Could you check a few things on this model? Use its own coordinates, in mm. A direction names the side the tool comes from. Round coordinates to 2 decimals unless told otherwise and drop trailing zeros. Loops run counter-clockwise (first coordinate to the right, second up) from the corner with the lowest first, then second, coordinate; pieces in that order, holes last. Notation, with made-up numbers: (61.5, -12) -> (113.5, -12) arc R8 cw to (113.5, 2) -> close; hole circle Ø3 at (77.5, -33.5). An arc over 180 degrees is marked (long way). One line per item, written item: value.
```python
from build123d import *

# Parameters (mm, degrees)
F0_W     = 50
F0_H     = 160
F0_R     = 3.25
F1_DEPTH = 5
F0_W_2   = 60
F2_DEPTH = 25


# Not quite as in the source:
# - a feature names something its author has since deleted; it is built from what else it names


with BuildPart() as f1:
    # F0 (on Front) → F1 (new body)
    with BuildSketch(Plane.XZ):
        with Locations((-52.5, 0)):
            Rectangle(F0_W, F0_H)
        with Locations((-47.5, -60)):
            Circle(F0_R, mode=Mode.SUBTRACT)
        with Locations((-47.5, 60)):
            Circle(F0_R, mode=Mode.SUBTRACT)
    extrude(amount=F1_DEPTH)



with BuildPart() as f1b:
    # F0 (on Front) → F1, piece 2 (new body)
    with BuildSketch(Plane.XZ):
        with Locations((57.5, 0)):
            Rectangle(F0_W, F0_H)
        with Locations((47.5, -60)):
            Circle(F0_R, mode=Mode.SUBTRACT)
        with Locations((47.5, 60)):
            Circle(F0_R, mode=Mode.SUBTRACT)
    extrude(amount=F1_DEPTH)


with BuildPart() as f1_1:
    add(f1.part)

    add(f1b.part)  # F2 merges F1b
    # F0 (on Front) → F2 (join)
    with BuildSketch(Plane.XZ):
        with Locations((2.5, 0)):
            Rectangle(F0_W_2, F0_H)
        with Locations((-17.5, -70)):
            Circle(F0_R, mode=Mode.SUBTRACT)
        with Locations((22.5, -70)):
            Circle(F0_R, mode=Mode.SUBTRACT)
        with Locations((-17.5, 70)):
            Circle(F0_R, mode=Mode.SUBTRACT)
        with Locations((22.5, 70)):
            Circle(F0_R, mode=Mode.SUBTRACT)
    extrude(amount=F2_DEPTH)


solid = f1_1.part
```
Item 1: For faces 4 (the face through (57, -5, 1)), 5 (the face through (-20.079, -12.325, -71.978)), 6 (the face through (-27.5, -15, -1)), which set-ups out of +Z, -Z, +X, -X, +Y, -Y let a thin tool reach every point of the face, with its end or its side?
Output:
face 4: +Z, -Z, +X, -Y
face 5: +Y, -Y
face 6: +Z, -Z, -X, -Y
Item 2: If we mould it in two halves opening along X, with no side actions, what happens to faces 1 (the face through (2, -25, 1)), 2 (the face through (-77.5, -2, -1)), 3 (the face through (-44.4, -2.46, 60.98))? For each: released by +X, released by -X, zero draft, split by the parting line, or undercut.
Output:
face 1: zero draft
face 2: released by -X
face 3: undercut
Item 3: If we section it at D-D on z = 10: List the corners of the cut face in (x, y) for me.
Output:
outline: (-77.5, -5) -> (-27.5, -5) -> (-27.5, -25) -> (32.5, -25) -> (32.5, -5) -> (82.5, -5) -> (82.5, 0) -> (-77.5, 0) -> close
Item 4: If we section it at C-C on x = 47.5: List the corners of the cut face in (y, z) for me, plus the area to 3 significant figures.
Output:
outline: (-5, -80) -> (0, -80) -> (0, -63.25) -> (-5, -63.25) -> close; (-5, -56.75) -> (0, -56.75) -> (0, 56.75) -> (-5, 56.75) -> close; (-5, 63.25) -> (0, 63.25) -> (0, 80) -> (-5, 80) -> close
area: 735 mm²
Item 5: I need wall thicknesses on line 1 (Z direction, x = -17.5, y = -17.75); line 2 (Z direction, x = 47.5, y = -1.9); line 3 (Y direction, x = -46, z = -30). Which ranges of each line are inside material? Lowest first, please. Write a range as from..to.
Output:
line 1: z = -80..-73.25, -66.75..66.75, 73.25..80
line 2: z = -80..-63.25, -56.75..56.75, 63.25..80
line 3: y = -5..0
Item 6: Will these pins go through, and if not, where does the flat tip stop? pin 1 Ø5 at (x, z) = (22.5, -70) entering from -Y; pin 2 Ø6 at (y, z) = (-18.5, 17.5) entering from -X; pin 3 Ø3 at (y, z) = (-10.5, -3.5) entering from +X; pin 4 Ø10.5 at (x, z) = (47.5, 60) entering from -Y.
Output:
pin 1: passes through
pin 2: stops at x = -27.5
pin 3: stops at x = 32.5
pin 4: stops at y = -5
Item 7: If we section it at A-A on z = 70: List the corners of the cut face in (x, y) for me.
Output:
outline: (-77.5, -5) -> (-27.5, -5) -> (-27.5, -25) -> (-20.75, -25) -> (-20.75, 0) -> (-77.5, 0) -> close; (-14.25, -25) -> (19.25, -25) -> (19.25, 0) -> (-14.25, 0) -> close; (25.75, -25) -> (32.5, -25) -> (32.5, -5) -> (82.5, -5) -> (82.5, 0) -> (25.75, 0) -> close
Item 8: If we section it at B-B on y = -11.25: List the corners of the cut face in (x, z) for me, plus the area to 3 significant figures.
Output:
outline: (-27.5, -80) -> (32.5, -80) -> (32.5, 80) -> (-27.5, 80) -> close; hole circle Ø6.5 at (-17.5, -70); hole circle Ø6.5 at (-17.5, 70); hole circle Ø6.5 at (22.5, -70); hole circle Ø6.5 at (22.5, 70)
area: 9,470 mm²
